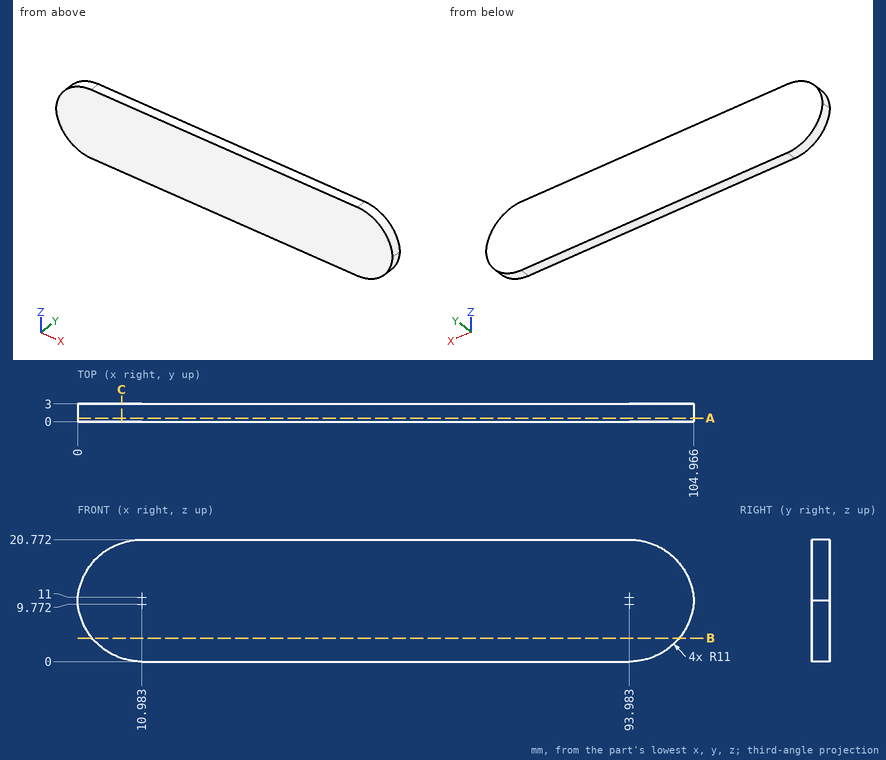
The figure shows three views and two pictorial views of one solid part (mm, origin at its lowest corner). Answer the questions. Coordinates: 2 decimals unless noted, no trailing zeros. Order: outer loops, then holes, each group sorted by start corner. A loop starts at its lowest first (then second) coordinate and runs counter-clockwise, first axis right, second up.
Q1. Given P1, Ø1, axis at x = 32, z = 15.5, coming from the -Y side; P2, Ø1, axis at y = 2.5, z = 4.5, coming from the +X side, each flat-ended and moving along its own axis, determine where each tip first touches the part or whether it passes through.
Q2. Consider line 1 (X direction, y = 1.35, z = 18.5) (1 decimal); line 2 (X direction, y = 2.25, z = 10.25); line 3 (Z direction, x = 100, y = 1). Determine where each line is inside the solid, lowest interval first.
Q3. A cutting plane is placed at C-C, the plane x = 7.5. Write down the section's boundary in (y, z).
Q4. A cutting plane is placed at B-B, the plane z = 4. Write down the section's boundary in (x, y), and give its area (3 significant figures).
Q5. A cutting plane is placed at A-A, the plane y = 0.6. Write down the section's boundary in (x, z) (1 decimal), and give its area (3 significant figures).
Answers follow:
1. P1: stops at y = 0
1. P2: stops at x = 103.2
2. line 1: x = 4.3 to 100.7
2. line 2: x = 0.01 to 104.96
2. line 3: z = 1.79 to 18.98
3. outline: (0, 0.57) - (3, 0.57) - (3, 20.21) - (0, 20.21) - close
4. outline: (2.5, 0) - (102.47, 0) - (102.47, 3) - (2.5, 3) - close
4. area: 300 mm2
5. outline: (0, 10.4) arc R11 ccw to (11, 0) - (94, 0) arc R11 ccw to (105, 10.4) arc R11 ccw to (94, 20.8) - (11, 20.8) arc R11 ccw to start
5. area: 2,080 mm2
